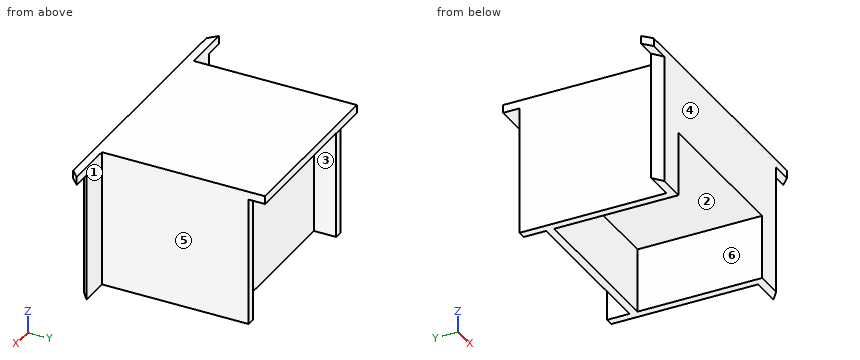
```python
from build123d import *

# Parameters (mm, degrees)
BOSS_EXTRUDE2_DEPTH = 50.8
SKETCH3_W           = 69.342
SKETCH3_H           = 67.437
BOSS_EXTRUDE3_DEPTH = 3.175
BOSS_EXTRUDE4_DEPTH = 53.975
BOSS_EXTRUDE6_DEPTH = 3.175
SKETCH6_W           = 62.992
SKETCH6_H           = 49.022
BOSS_EXTRUDE7_DEPTH = 25.4


with BuildPart() as part:
    # Sketch2 → Boss-Extrude2 (new body)
    with BuildSketch(Plane.XY):
        Polygon((-34.671, -49.022), (-31.496, -49.022), (-31.496, 0), (31.496, 0), (31.496, -49.022), (34.671, -49.022), (34.671, 11.938), (31.496, 11.938), (31.496, 3.175), (-31.496, 3.175), (-31.496, 11.938), (-34.671, 11.938), align=None)
    extrude(amount=BOSS_EXTRUDE2_DEPTH)

    # Sketch3 → Boss-Extrude3 (add)
    with BuildSketch(Plane.XY.offset(50.8)):
        with Locations((0, -15.3035)):
            Rectangle(SKETCH3_W, SKETCH3_H)
    extrude(amount=BOSS_EXTRUDE3_DEPTH)

    # Sketch4 → Boss-Extrude4 (add)
    with BuildSketch(Plane.XY.offset(53.975)):
        with BuildLine():
            Line((-34.671, -49.022), (-42.1386, -49.022))
            ThreePointArc((-42.1386, -49.022), (-44.170473584, -47.470511893), (-46.145273507, -45.847))
            Line((-46.145273507, -45.847), (-34.671, -45.847))
            Line((-34.671, -45.847), (-34.671, -49.022))
        make_face()
        with BuildLine():
            Line((34.671, -45.847), (34.671, -49.022))
            Line((34.671, -49.022), (42.1386, -49.022))
            ThreePointArc((42.1386, -49.022), (44.170473584, -47.470511893), (46.145273507, -45.847))
            Line((46.145273507, -45.847), (34.671, -45.847))
        make_face()
    extrude(amount=-BOSS_EXTRUDE4_DEPTH)

    # Sketch5 → Boss-Extrude6 (add)
    with BuildSketch(Plane(origin=(0, 0, 53.975), x_dir=(-1, 0, 0), z_dir=(0, 0, -1))):
        with BuildLine():
            Line((42.1386, -49.022), (50.239896596, -49.022))
            ThreePointArc((50.239896596, -49.022), (51.966635807, -47.460510217), (53.64486804, -45.847))
            Line((53.64486804, -45.847), (46.145273507, -45.847))
            ThreePointArc((46.145273507, -45.847), (44.170473584, -47.470511893), (42.1386, -49.022))
        make_face()
        with BuildLine():
            Line((-46.145273507, -45.847), (-53.64486804, -45.847))
            ThreePointArc((-53.64486804, -45.847), (-51.966635807, -47.460510217), (-50.239896596, -49.022))
            Line((-50.239896596, -49.022), (-42.1386, -49.022))
            ThreePointArc((-42.1386, -49.022), (-44.170473584, -47.470511893), (-46.145273507, -45.847))
        make_face()
    extrude(amount=BOSS_EXTRUDE6_DEPTH)

    # Sketch6 → Boss-Extrude7 (add)
    with BuildSketch(Plane(origin=(0, 0, 50.8), x_dir=(-1, 0, 0), z_dir=(0, 0, -1))):
        with Locations((0, -24.511)):
            Rectangle(SKETCH6_W, SKETCH6_H)
    extrude(amount=BOSS_EXTRUDE7_DEPTH)


solid = part.part
```
The model under review builds one solid part; all positions refer to its coordinate system, in mm. Face numbers are marked on the shaded views. A direction names the side the tool comes from. Round coordinates to 2 decimals unless told otherwise and drop trailing zeros. Write each loop counter-clockwise with the first axis right and the second up, starting at its lowest first coordinate (ties: lowest second). Pieces come first, ordered by that corner, then holes. Notation, with made-up numbers: (43, 28) - (91, 28) arc R15 cw to (91, 45) - close; hole circle Ø4 at (-30.75, -23.5). An arc over 180 degrees is marked (long way). Answer as CSV lines item,"result". Start each with the question number.
(1) We need section C-C on y = -38. State the section outline as (x, z) points (3 decimals), plus the area to 3 significant figures.
(2) To check wall thickness, follow line 1 (X direction, y = -7, z = 20); line 2 (X direction, y = -35, z = 30); line 3 (Z direction, x = -25.5, y = 5.5) (3 decimals). State the ranges of each line that lie inside material, in increasing order.
(3) For pin 1 Ø5.5 at (x, z) = (45, 40.5) entering from +Y; pin 2 Ø24.5 at (x, y) = (-11, -24.5) entering from -Z; pin 3 Ø3 at (y, z) = (-36, 39.5) entering from +X, all flat-tipped, find the tip position at first contact; note any pin that passes through.
(4) For the marked faces 1, 2 and 3, list the 3-axis set-ups (+Z, -Z, +X, -X, +Y, -Y) from which the entire face can be reached by the end or side of a thin tool; tool diameter is ignored.
(5) Draft analysis for pull direction X (two halves, no side actions). For the marked faces 4, 5 and 6, state which applies: pulls with the +X half, pulls with the -X half, needs draft (parallel to the pull), parting line crosses it, or undercut.
(6) We need section B-B on x = 16. State the section outline as (y, z) points (3 decimals).
(7) We need section A-A on z = 43. State the section outline as (x, y) points (3 decimals), plus the area to 3 significant figures.
(8) We need section D-D on z = 16. State the section outline as (x, y) points (3 decimals).
Worked answers:
1,outline,"(-34.671, 0) - (-31.496, 0) - (-31.496, 25.4) - (31.496, 25.4) - (31.496, 0) - (34.671, 0) - (34.671, 53.975) - (-34.671, 53.975) - close"
1,area,"2,140 mm²"
2,line 1,"-34.67 to -31.5, 31.5 to 34.67"
2,line 2,"-34.67 to 34.67"
2,line 3,"50.8 to 53.975"
3,pin 1,"y = -45.85"
3,pin 2,"z = 25.4"
3,pin 3,"x = 34.67"
4,face 1,"+Z, -Z, +X, +Y"
4,face 2,"-Z, -Y"
4,face 3,"-Z, +Y"
5,face 4,"needs draft"
5,face 5,"pulls with the +X half"
5,face 6,"undercut"
6,outline,"(-49.022, 25.4) - (0, 25.4) - (0, 0) - (3.175, 0) - (3.175, 50.8) - (18.415, 50.8) - (18.415, 53.975) - (-49.022, 53.975) - close"
7,outline,"(-46.145, -45.847) arc R71.12 ccw to (-42.139, -49.022) - (42.139, -49.022) arc R71.12 ccw to (46.145, -45.847) - (34.671, -45.847) - (34.671, 11.938) - (31.496, 11.938) - (31.496, 3.175) - (-31.496, 3.175) - (-31.496, 11.938) - (-34.671, 11.938) - (-34.671, -45.847) - close"
7,area,"3,740 mm²"
8,outline,"(-46.145, -45.847) arc R71.12 ccw to (-42.139, -49.022) - (-31.496, -49.022) - (-31.496, 0) - (31.496, 0) - (31.496, -49.022) - (42.139, -49.022) arc R71.12 ccw to (46.145, -45.847) - (34.671, -45.847) - (34.671, 11.938) - (31.496, 11.938) - (31.496, 3.175) - (-31.496, 3.175) - (-31.496, 11.938) - (-34.671, 11.938) - (-34.671, -45.847) - close"
